Source: three-view drawing plus pictorial views. Frame: mm from the lowest corner of the part. Round coordinates to 2 decimals unless told otherwise and drop trailing zeros. Order: outer loops, then holes, each group sorted by start corner. A loop starts at its lowest first (then second) coordinate and runs counter-clockwise, first axis right, second up. Notation, with made-up numbers: (13.25, 57.25) - (29.25, 57.25) arc R23 ccw to (29.25, 70.25) - close; hole circle Ø4 at (-34.5, -30). An arc over 180 degrees is marked (long way). Use one line per item in the form item = value. Start each with the question number.
Q1. Pin query (flat end, axial travel): pin 1 Ø3 at (x, z) = (18.5, 3) entering from +Y. Return the tip coordinate at first contact, or that it passes through.
Q2. Ray query, line 1 (Z direction, x = 66, y = 1.3); line 2 (X direction, y = 1, z = 0.7); line 3 (Z direction, x = 83.5, y = 1.5). Return the intervals inside material, ascending. Write a range as [from, to].
Q3. Cut plane A-A, the plane x = 82. Return the cut outline in (y, z).
Q4. Cut plane B-B, the plane y = 2.4. Give the number of separate pieces and of enclosed holes in the cut face, and give its area (3 significant figures).
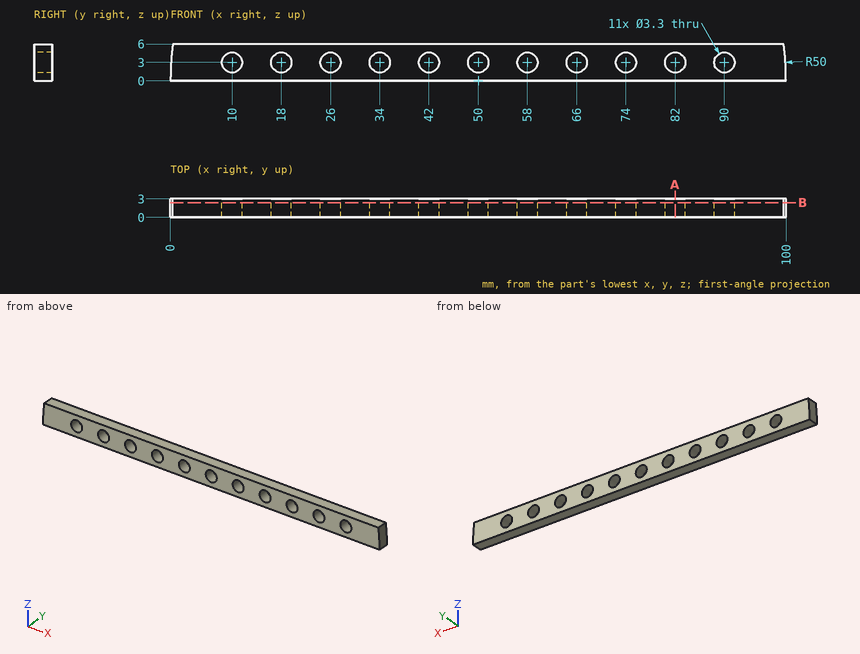
Completed:
q1.pin_1 = 3
q2.line_1 = [0, 1.35], [4.65, 6]
q2.line_2 = [0, 100]
q2.line_3 = [0, 2.31], [3.69, 6]
q3.outline = (0, 0) - (3, 0) - (3, 1.35) - (0, 1.35) - close; (0, 4.65) - (3, 4.65) - (3, 6) - (0, 6) - close
q4.separate_pieces = 1
q4.enclosed_holes = 11
q4.area = 504 mm2
